The listing builds one solid part. Answer for the finished solid, in the listing's coordinates (mm). A direction names the side the tool comes from. Give positions to 0.01 mm unless a question says otherwise; leave off trailing zeros. Order: outer loops, then holes, each group sorted by start corner. A loop starts at its lowest first (then second) coordinate and runs counter-clockwise, first axis right, second up. Notation, with made-up numbers: (50, -37.75) - (72, -37.75) arc R18 cw to (72, -10.75) - close; hole circle Ø4 at (-27, -0.5). An arc over 180 degrees is marked (long way). Answer in a Markdown table with one row per item.
from build123d import *

# Parameters (mm, degrees)
EXTRUDE_1_DEPTH = 3


with BuildPart() as part:
    # 草图1 → 凸台-拉伸1 (new body)
    with BuildSketch(Plane.XY):
        Polygon((277.453360513, -198.037068397), (277.453360513, -203.037068397), (222.453360513, -203.037068397), (222.453360513, -198.037068397), (224.953360513, -198.037068397), (224.953360513, -199.537068397), (227.553360513, -199.537068397), (227.553360513, -198.037068397), (230.553360513, -198.037068397), (230.553360513, -195.037068397), (227.553360513, -195.037068397), (227.553360513, -193.537068397), (224.953360513, -193.537068397), (224.953360513, -195.037068397), (222.453360513, -195.037068397), (222.453360513, -144.126812717), (219.453360513, -144.126812717), (219.453360513, -140.126812717), (219.453360513, -136.126812717), (222.453360513, -136.126812717), (222.453360513, -85.216557036), (224.953360513, -85.216557036), (224.953360513, -86.716557036), (227.553360513, -86.716557036), (227.553360513, -85.216557036), (230.553360513, -85.216557036), (230.553360513, -82.216557036), (227.553360513, -82.216557036), (227.553360513, -80.716557036), (224.953360513, -80.716557036), (224.953360513, -82.216557036), (222.453360513, -82.216557036), (222.453360513, 78.373187283), (219.453360513, 78.373187283), (219.453360513, 82.373187283), (219.453360513, 86.373187283), (222.453360513, 86.373187283), (222.453360513, 246.962931603), (224.953360513, 246.962931603), (224.953360513, 245.462931603), (227.553360513, 245.462931603), (227.553360513, 246.962931603), (230.553360513, 246.962931603), (230.553360513, 249.962931603), (227.553360513, 249.962931603), (227.553360513, 251.462931603), (224.953360513, 251.462931603), (224.953360513, 249.962931603), (222.453360513, 249.962931603), (222.453360513, 254.962931603), (277.453360513, 254.962931603), (277.453360513, 249.962931603), (274.953360513, 249.962931603), (274.953360513, 251.462931603), (272.353360513, 251.462931603), (272.353360513, 249.962931603), (269.353360513, 249.962931603), (269.353360513, 246.962931603), (272.353360513, 246.962931603), (272.353360513, 245.462931603), (274.953360513, 245.462931603), (274.953360513, 246.962931603), (277.453360513, 246.962931603), (277.453360513, 196.052675922), (280.453360513, 196.052675922), (280.453360513, 192.052675922), (280.453360513, 188.052675922), (277.453360513, 188.052675922), (277.453360513, 137.142420241), (274.953360513, 137.142420241), (274.953360513, 138.642420241), (272.353360513, 138.642420241), (272.353360513, 137.142420241), (269.353360513, 137.142420241), (269.353360513, 134.142420241), (272.353360513, 134.142420241), (272.353360513, 132.642420241), (274.953360513, 132.642420241), (274.953360513, 134.142420241), (277.453360513, 134.142420241), (277.453360513, -26.447324078), (280.453360513, -26.447324078), (280.453360513, -30.447324078), (280.453360513, -34.447324078), (277.453360513, -34.447324078), (277.453360513, -195.037068397), (274.953360513, -195.037068397), (274.953360513, -193.537068397), (272.353360513, -193.537068397), (272.353360513, -195.037068397), (269.353360513, -195.037068397), (269.353360513, -198.037068397), (272.353360513, -198.037068397), (272.353360513, -199.537068397), (274.953360513, -199.537068397), (274.953360513, -198.037068397), align=None)
        with BuildLine():
            Line((233.453360513, 232.962931603), (265.776162867, 232.962931603))
            ThreePointArc((265.776162867, 232.962931603), (268.007619579, 231.968075224), (268.759090329, 229.643332232))
            Line((268.759090329, 229.643332232), (236.436287975, -72.036156407))
            ThreePointArc((236.436287975, -72.036156407), (233.293332993, -74.712285861), (230.453360513, -71.716557036))
            Line((230.453360513, -71.716557036), (230.453360513, 229.962931603))
            ThreePointArc((230.453360513, 229.962931603), (231.33204017, 232.084251946), (233.453360513, 232.962931603))
        make_face(mode=Mode.SUBTRACT)
        with BuildLine():
            Line((269.453360513, 123.642420241), (269.453360513, -178.037068397))
            ThreePointArc((269.453360513, -178.037068397), (268.574680857, -180.158388741), (266.453360513, -181.037068397))
            Line((266.453360513, -181.037068397), (234.130558159, -181.037068397))
            ThreePointArc((234.130558159, -181.037068397), (231.899101447, -180.042212019), (231.147630697, -177.717469026))
            Line((231.147630697, -177.717469026), (263.470433052, 123.962019612))
            ThreePointArc((263.470433052, 123.962019612), (266.613388034, 126.638149066), (269.453360513, 123.642420241))
        make_face(mode=Mode.SUBTRACT)
    extrude(amount=EXTRUDE_1_DEPTH)


solid = part.part
Item 1: Each of these flat-tipped pins is pushed along its axis until it touches: P1, Ø0.8, axis at y = -198.5, z = 1, coming from the +X side; P2, Ø1.2, axis at y = -194, z = 1.5, coming from the -X side; P3, Ø1.5, axis at y = 249, z = 1.5, coming from the +X side. Where does it stop, or does it pass through?
Answer block:
| item | result |
|---|---|
| P1 | x = 277.45 |
| P2 | x = 222.45 |
| P3 | x = 269.35 |
Item 2: Find section B-B on x = 250.5. Write down the section's boundary in (y, z), then the cut area to 3 significant figures.
Answer block:
| item | result |
|---|---|
| outline | (-203.04, 0) - (-181.04, 0) - (-181.04, 3) - (-203.04, 3) - close; (2.9, 0) - (59.23, 0) - (59.23, 3) - (2.9, 3) - close; (232.96, 0) - (254.96, 0) - (254.96, 3) - (232.96, 3) - close |
| area | 301 mm² |
Item 3: Determine the mould class of faces 3 (the face through (250, 29, 3)), 4 (the face through (252.824, 80.915, 1.479)) for opening direction X: pulls with the +X half, pulls with the -X half, needs draft (parallel to the pull), parting line crosses it, or undercut.
Answer block:
| item | result |
|---|---|
| face 3 | needs draft |
| face 4 | undercut |
Item 4: Consider line 1 (Y direction, x = 224, z = 2.55); line 2 (Y direction, x = 273, z = 2.4); line 3 (X direction, y = -26, z = 1). Determine where each line is inside the solid, lowest interval first.
Answer block:
| item | result |
|---|---|
| line 1 | -203.04 to -198.04, -195.04 to -85.22, -82.22 to 246.96, 249.96 to 254.96 |
| line 2 | -203.04 to -199.54, -193.54 to 132.64, 138.64 to 245.46, 251.46 to 254.96 |
| line 3 | 222.45 to 230.45, 241.37 to 247.4, 269.45 to 277.45 |
Item 5: Find section A-A on y = 118.5. Write down the section's boundary in (x, z).
Answer block:
| item | result |
|---|---|
| outline | (222.45, 0) - (230.45, 0) - (230.45, 3) - (222.45, 3) - close; (256.85, 0) - (262.89, 0) - (262.89, 3) - (256.85, 3) - close; (269.45, 0) - (277.45, 0) - (277.45, 3) - (269.45, 3) - close |
Item 6: Which of the six approach directions +Z, -Z, +X, -X, +Y, -Y give full straight-line access (tool end or side, diameter ignored) to faces 1 (the face through (250, 29, 0)), 2 (the face through (247.083, -28.989, 1.479))?
Answer block:
| item | result |
|---|---|
| face 1 | -Z, +X, -X, +Y, -Y |
| face 2 | +Z, -Z |
Item 7: Find section C-C on z = 2.15. Count the separate pieces of the cut face and the enclosed holes in it, then the cut area to 3 significant figures.
Answer block:
| item | result |
|---|---|
| separate pieces | 1 |
| enclosed holes | 2 |
| area | 11,500 mm² |
